```python
from build123d import *

# Parameters (mm, degrees)
SKETCH6_W           = 34.925
SKETCH6_H           = 5.55625
EXTRUDE1_DEPTH      = 8.00608
SKETCH7_W           = 34.925
SKETCH7_H           = 2.1844
SKETCH17_R          = 5.55625
CUT_EXTRUDE1_DEPTH  = 12.63142
SKETCH19_R          = 6.858
BOSS_EXTRUDE1_DEPTH = 12.63142
BOSS_EXTRUDE1_DRAFT = -1.75
CHAMFER1_SIZE       = 1.058333333
CHAMFER1_SIZE2      = 1.092196811
SKETCH22_R          = 6.858
BOSS_EXTRUDE3_DEPTH = 12.63142
BOSS_EXTRUDE3_DRAFT = -15
SKETCH23_R          = 4.651741881
CUT_EXTRUDE2_DEPTH  = 12.63142


with BuildPart() as part:
    # Sketch6 → Revolve3 (revolve)
    with BuildSketch(Plane.XY, mode=Mode.PRIVATE) as revolve3_sk:
        with Locations((0, 2.778125)):
            Rectangle(SKETCH6_W, SKETCH6_H)
    revolve(revolve3_sk.sketch.rotate(Axis((-17.4625, 0, 0), (1, 0, 0)), 90), axis=Axis((-17.4625, 0, 0), (1, 0, 0)))

    # Sketch12 → Extrude1 (add)
    with BuildSketch(Plane(origin=(-4.83108, 0, 0), x_dir=(0, 0, -1), z_dir=(1, 0, 0))):
        Polygon((0, 8.248891971), (-7.14375, 4.124445986), (-7.14375, -4.124445986), (0, -8.248891971), (7.14375, -4.124445986), (7.14375, 4.124445986), align=None)
    extrude(amount=EXTRUDE1_DEPTH)

    # Sketch10 → Cut-Revolve6 (revolve, cut)
    with BuildSketch(Plane.XY, mode=Mode.PRIVATE) as cut_revolve6_sk:
        Polygon((5.003189197, 5.55625), (3.175, 5.55625), (3.175, 4.680560803), (4.1275, 4.680560803), align=None)
        Polygon((17.4625, 5.55625), (11.804113042, 5.55625), (12.679802239, 4.680560803), (14.584802239, 4.680560803), (17.4625, 2.51206), align=None)
    revolve(cut_revolve6_sk.sketch.rotate(Axis((-17.4625, 0, 0), (1, 0, 0)), 90), axis=Axis((-17.4625, 0, 0), (1, 0, 0)), mode=Mode.SUBTRACT)

    # Sketch7 → Cut-Revolve5 (revolve, cut)
    with BuildSketch(Plane.XY):
        with Locations((0, 1.0922)):
            Rectangle(SKETCH7_W, SKETCH7_H)
    revolve(axis=Axis((17.4625, 0, 0), (-1, 0, 0)), mode=Mode.SUBTRACT)

    # Sketch13 → Cut-Revolve7 (revolve, cut)
    with BuildSketch(Plane.XY):
        Polygon((-4.83108, 8.248891971), (-4.83108, 7.14375), (-4.193025986, 8.248891971), align=None)
        Polygon((2.536945986, 8.248891971), (3.175, 7.14375), (3.175, 8.248891971), align=None)
    revolve(axis=Axis((-17.4625, 0, 0), (1, 0, 0)), mode=Mode.SUBTRACT)

    # Sketch17 → Cut-Extrude1 (cut)
    with BuildSketch(Plane.ZY.offset(17.4625)):
        Circle(SKETCH17_R)
    extrude(amount=-CUT_EXTRUDE1_DEPTH, mode=Mode.SUBTRACT)


with BuildPart() as body_2:
    # Sketch19 → Boss-Extrude1 (with draft: the straight prism first)
    with BuildSketch(Plane(origin=(-4.83108, 0, 0), x_dir=(0, 0, -1), z_dir=(1, 0, 0))):
        Circle(SKETCH19_R)
    extrude(amount=-BOSS_EXTRUDE1_DEPTH)
    # Boss-Extrude1: the draft: its side faces are tilted about the plane it starts from
    boss_extrude1_sides = [body_2.faces().sort_by_distance(p)[0] for p in [
        (-11.14679, 0, 6.858),
    ]]
    draft(boss_extrude1_sides, Plane(origin=(-4.83108, 0, 0), x_dir=(0, 0, -1), z_dir=(1, 0, 0)), BOSS_EXTRUDE1_DRAFT)

    # Chamfer1
    chamfer1_edges = [body_2.edges().sort_by_distance(p)[0] for p in [
        (-17.4625, 0, 6.472075215),
    ]]
    chamfer1_side = [body_2.faces().sort_by_distance(p)[0] for p in [
        (-17.4625, 0, 0),
    ]]
    chamfer(chamfer1_edges, length=CHAMFER1_SIZE, length2=CHAMFER1_SIZE2, reference=chamfer1_side[0])


with BuildPart() as boss_extrude3_tool:
    # Sketch22 → Boss-Extrude3 (with draft: the straight prism first)
    with BuildSketch(Plane(origin=(-4.83108, 0, 0), x_dir=(0, 0, -1), z_dir=(1, 0, 0))):
        Circle(SKETCH22_R)
    extrude(amount=-BOSS_EXTRUDE3_DEPTH)
    # Boss-Extrude3: the draft: its side faces are tilted about the plane it starts from
    boss_extrude3_sides = [boss_extrude3_tool.faces().sort_by_distance(p)[0] for p in [
        (-11.14679, 0, 6.858),
    ]]
    draft(boss_extrude3_sides, Plane(origin=(-4.83108, 0, 0), x_dir=(0, 0, -1), z_dir=(1, 0, 0)), BOSS_EXTRUDE3_DRAFT)


with BuildPart() as body_2_1:
    add(body_2.part)

    # Boss-Extrude3: add boss_extrude3_tool
    add(boss_extrude3_tool.part)

    # Combine1: union part
    add(part.part)

    # Sketch23 → Cut-Extrude2 (cut)
    with BuildSketch(Plane.ZY.offset(17.4625)):
        Circle(SKETCH23_R)
    extrude(amount=-CUT_EXTRUDE2_DEPTH, mode=Mode.SUBTRACT)


solid = body_2_1.part
```
Read the model definition and answer for the solid it produces. Units are mm, in the model's axes. A direction names the side the tool comes from. Coordinates: 2 decimals unless noted, no trailing zeros. Write each loop counter-clockwise with the first axis right and the second up, starting at its lowest first coordinate (ties: lowest second). Pieces come first, ordered by that corner, then holes. Notation, with made-up numbers: (62.5, 10) - (77.5, 10) arc R16 cw to (77.5, 34) - close; hole circle Ø2 at (-32, -21). An arc over 180 degrees is marked (long way). Answer as a JSON object with one key per item and string values. Group by question number.
1. Each of these flat-tipped pins is pushed along its axis until it touches: P1, Ø3, axis at x = -8.5, z = -4, coming from the +Y side; P2, Ø1.5, axis at y = -5, z = 4, coming from the +X side (3 decimals); P3, Ø1, axis at y = -2, z = 2, coming from the -X side; P4, Ø2.5, axis at y = 0, z = 0, coming from the +X side. Where does it stop, or does it pass through?
2. Consider L1, parallel to Y at x = 8.25, z = 0; L2, parallel to Y at x = 13.25, z = 0; L3, parallel to Z at x = -12, y = 4. Determine where each line is inside the solid, lowest interval first. Write a range as [from, to].
3. A cutting plane is placed at B-B (x = 7.5). Determine the outline of the cut face in (y, z), plus the area to 3 significant figures.
4. Which of the six approach directions +Z, -Z, +X, -X, +Y, -Y give full straight-line access (tool end or side, diameter ignored) to faces 1 (the conical face through (-10.52, -6.525, 1.449)), 2 (the conical face through (-4.676, 3.722, 6.41))?
5. The mould has two halves that part along Y. Classify faces 3 (the flat face through (-4.831, -0.97, -2.13)), 4 (the conical face through (17.323, 2.555, -0.567)), 5 (the conical face through (-4.676, 7.412, -0.018)): +Y half, -Y half, draft (parallel to the pull), parting line (faces both ways), or undercut.
6. A cutting plane is placed at A-A (x = 1.5). Determine the outline of the cut face in (y, z), plus the area to 3 significant figures.
Worked out:
{
 "1": {"P1": "stops at y = 6.27", "P2": "stops at x = 3.175", "P3": "stops at x = -4.83", "P4": "passes through"},
 "2": {"L1": "y = [-5.56, -2.18], [2.18, 5.56]", "L2": "y = [-4.68, -2.18], [2.18, 4.68]", "L3": "z = [-5.3, -2.37], [2.37, 5.3]"},
 "3": {"outline": "circle Ø11.11 at (0, 0); hole circle Ø4.37 at (0, 0)", "area": "82.0 mm²"},
 "4": {"face 1": "-X", "face 2": "+Z, -X, +Y"},
 "5": {"face 3": "undercut", "face 4": "parting line", "face 5": "+Y half"},
 "6": {"outline": "(-8.25, 0) - (-4.12, -7.14) - (4.12, -7.14) - (8.25, 0) - (4.12, 7.14) - (-4.12, 7.14) - close; hole circle Ø4.37 at (0, 0)", "area": "162 mm²"}
}
